For this review, take the finished solid that the model builds, in its own axes (mm). Coordinates: 2 decimals unless noted, no trailing zeros. Write each loop counter-clockwise with the first axis right and the second up, starting at its lowest first coordinate (ties: lowest second). Pieces come first, ordered by that corner, then holes.
1) We need section B-B on y = -64. Write out the cut boundary in (x, z).
2) We need section C-C on x = 131. Write out the cut boundary in (y, z), then the cut area to 3 significant figures.
3) To check wall thickness, follow line 1 along X through (y, z) = (-42.5, 1.9); line 2 along Y through (x, z) = (45.5, 3.05); line 3 along X through (y, z) = (-58.5, 3.45). State the ranges of each line that lie inside material, in increasing order.
4) Insertion check: P1, Ø1.2, axis at y = 2, z = 1.5, coming from the +X side; P2, Ø2, axis at x = 44, z = 2, coming from the +Y side; P3, Ø1, axis at x = 53, y = -18.5, coming from the -Z side; P4, Ø2, axis at y = 2.5, z = 1.5, coming from the -X side. Each pin has a flat end and moves straight along its axis. Give the tip position at first contact, or say it passes through.
5) We need section A-A on x = 45.5. Write out the cut boundary in (y, z).
from build123d import *

# Parameters (mm, degrees)
BOSS_EXTRUDE1_DEPTH = 4.064
SKETCH2_W           = 4.064
SKETCH2_H           = 12.7
CUT_EXTRUDE1_DEPTH  = 5.064
CUT_EXTRUDE2_DEPTH  = 5.064


with BuildPart() as part:
    # Sketch1 → Boss-Extrude1 (new body)
    with BuildSketch(Plane.XY):
        Polygon((-118.4275, -120.65), (-118.4275, -97.663), (118.4275, -97.663), (118.4275, -120.65), (223.0755, -120.65), (223.0755, 0), (197.6755, 0), (197.6755, 4.064), (178.6255, 4.064), (178.6255, 0), (-178.6255, 0), (-178.6255, 4.064), (-197.6755, 4.064), (-197.6755, 0), (-223.0755, 0), (-223.0755, -120.65), align=None)
    extrude(amount=BOSS_EXTRUDE1_DEPTH)

    # Sketch2 → Cut-Extrude1 (cut, through all)
    with BuildSketch(Plane.XY.offset(4.064)):
        with Locations((-221.0435, -38.1)):
            Rectangle(SKETCH2_W, SKETCH2_H)
        with Locations((-221.0435, -95.25)):
            Rectangle(SKETCH2_W, SKETCH2_H)
        with Locations((221.0435, -95.25)):
            Rectangle(SKETCH2_W, SKETCH2_H)
        with Locations((221.0435, -38.1)):
            Rectangle(SKETCH2_W, SKETCH2_H)
    extrude(amount=-CUT_EXTRUDE1_DEPTH, mode=Mode.SUBTRACT)

    # Sketch3 → Cut-Extrude2 (cut, through all)
    with BuildSketch(Plane.XY.offset(4.064)):
        with BuildLine():
            Line((-93.0275, -19.05), (93.0275, -19.05))
            ThreePointArc((93.0275, -19.05), (102.007756121, -22.769743879), (105.7275, -31.75))
            Line((105.7275, -31.75), (105.7275, -59.563))
            ThreePointArc((105.7275, -59.563), (102.007756121, -68.543256121), (93.0275, -72.263))
            Line((93.0275, -72.263), (-93.0275, -72.263))
            ThreePointArc((-93.0275, -72.263), (-102.007756121, -68.543256121), (-105.7275, -59.563))
            Line((-105.7275, -59.563), (-105.7275, -31.75))
            ThreePointArc((-105.7275, -31.75), (-102.007756121, -22.769743879), (-93.0275, -19.05))
        make_face()
    extrude(amount=-CUT_EXTRUDE2_DEPTH, mode=Mode.SUBTRACT)


solid = part.part
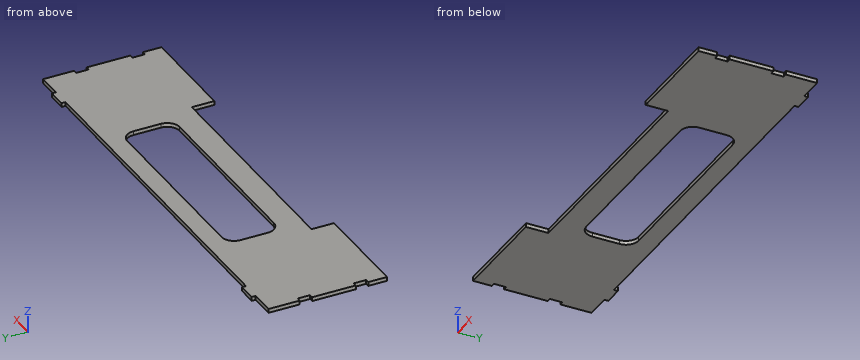
Result:
1. outline: (-223.08, 0) - (-104.93, 0) - (-104.93, 4.06) - (-223.08, 4.06) - close; (104.93, 0) - (223.08, 0) - (223.08, 4.06) - (104.93, 4.06) - close
2. outline: (-120.65, 0) - (0, 0) - (0, 4.06) - (-120.65, 4.06) - close
2. area: 490 mm2
3. line 1: x = -219.01 to -105.73, 105.73 to 219.01
3. line 2: y = -97.66 to -72.26, -19.05 to 0
3. line 3: x = -223.08 to -105.73, 105.73 to 223.08
4. P1: stops at x = 197.68
4. P2: stops at y = 0
4. P3: stops at z = 0
4. P4: stops at x = -197.68
5. outline: (-97.66, 0) - (-72.26, 0) - (-72.26, 4.06) - (-97.66, 4.06) - close; (-19.05, 0) - (0, 0) - (0, 4.06) - (-19.05, 4.06) - close
